from build123d import *

# Parameters (mm, degrees)
SKETCH_W        = 23
SKETCH_H        = 12
PAD_DEPTH       = 1
SKETCH001_W     = 4
SKETCH001_H     = 4
SKETCH001_W_2   = 9
SKETCH001_W_3   = 1.8
SKETCH001_H_2   = 2.119738
SKETCH001_W_4   = 1.7
SKETCH001_H_3   = 1.880262
SKETCH001_H_4   = 2.108956
SKETCH001_W_5   = 1.95
SKETCH001_H_5   = 1.880263
SKETCH001_H_6   = 2.119737
POCKET_DEPTH    = 5
SKETCH002_W     = 6
SKETCH002_H     = 12
POCKET001_DEPTH = 5


with BuildPart() as part:
    # Sketch → Pad (new body)
    with BuildSketch(Plane.XZ):
        with Locations((0.224666, -4.175566)):
            Rectangle(SKETCH_W, SKETCH_H)
    extrude(amount=PAD_DEPTH)

    # Sketch001 (on Face6 of Pad) → Pocket (cut)
    with BuildSketch(Plane.XZ.offset(1)):
        with Locations((-7.275334, -6.675566)):
            Rectangle(SKETCH001_W, SKETCH001_H)
        with Locations((7.724666, -6.675566)):
            Rectangle(SKETCH001_W, SKETCH001_H)
        with Locations((0.224666, -6.675566)):
            Rectangle(SKETCH001_W_2, SKETCH001_H)
        with Locations((-8.375334, -0.735435)):
            Rectangle(SKETCH001_W_3, SKETCH001_H_2)
        with Locations((-6.125334, -0.735435)):
            Rectangle(SKETCH001_W_4, SKETCH001_H_2)
        with Locations((-8.375334, -3.235435)):
            Rectangle(SKETCH001_W_3, SKETCH001_H_3)
        with Locations((-6.125334, -3.235435)):
            Rectangle(SKETCH001_W_4, SKETCH001_H_3)
        with Locations((-3.375334, -0.730044)):
            Rectangle(SKETCH001_W_3, SKETCH001_H_4)
        with Locations((-1.000334, -0.730044)):
            Rectangle(SKETCH001_W_5, SKETCH001_H_4)
        with Locations((-3.375334, -3.224654)):
            Rectangle(SKETCH001_W_3, SKETCH001_H_5)
        with Locations((-1.000334, -3.224654)):
            Rectangle(SKETCH001_W_5, SKETCH001_H_5)
        with Locations((1.374666, -0.730044)):
            Rectangle(SKETCH001_W_3, SKETCH001_H_4)
        with Locations((3.674666, -0.724653)):
            Rectangle(SKETCH001_W_3, SKETCH001_H_6)
        with Locations((1.374666, -3.224654)):
            Rectangle(SKETCH001_W_3, SKETCH001_H_5)
        with Locations((3.749666, -3.224654)):
            Rectangle(SKETCH001_W_5, SKETCH001_H_5)
        with Locations((6.624666, -0.732224)):
            Rectangle(SKETCH001_W_3, SKETCH001_H_2)
        with Locations((8.874666, -0.732224)):
            Rectangle(SKETCH001_W_4, SKETCH001_H_2)
        with Locations((6.624666, -3.232224)):
            Rectangle(SKETCH001_W_3, SKETCH001_H_3)
        with Locations((8.874666, -3.232224)):
            Rectangle(SKETCH001_W_4, SKETCH001_H_3)
    extrude(amount=-POCKET_DEPTH, mode=Mode.SUBTRACT)

    # Sketch002 (on Face5 of Pocket) → Pocket001 (cut)
    with BuildSketch(Plane.XZ.offset(1)):
        with Locations((-8.275334, -4.175566)):
            Rectangle(SKETCH002_W, SKETCH002_H)
        with Locations((8.724666, -4.175566)):
            Rectangle(SKETCH002_W, SKETCH002_H)
    extrude(amount=-POCKET001_DEPTH, mode=Mode.SUBTRACT)


solid = part.part
Work out the finished part from the listing and answer in its coordinate system (mm). A direction names the side the tool comes from. Round coordinates to 2 decimals unless told otherwise and drop trailing zeros. Write each loop counter-clockwise with the first axis right and the second up, starting at its lowest first coordinate (ties: lowest second). Pieces come first, ordered by that corner, then holes.
1) A cutting plane is placed at A-A (z = -2.75). Give the vertices of the cut face in (x, y).
2) A cutting plane is placed at D-D (z = -1). Give the vertices of the cut face in (x, y).
3) A tool of negligible diameter and unlimited length cuts with its end or side. For faces 3 (the flat face through (2.275, -0.5, -0.7)), 4 (the flat face through (5.725, -0.5, -4.3)), from which of +Z, -Z, +X, -X, +Y, -Y can it reach the whole face along a straight path? Write none if from no direction.
4) A cutting plane is placed at C-C (x = 1). Give the vertices of the cut face in (y, z).
5) Straight lines are drawn through the part: line 1 (X direction, y = -0.55, z = -2.75); line 2 (Z direction, x = 3.75, y = -0.85); line 3 (X direction, y = -0.35, z = -1.75). For each, find the intervals that lie inside material, in ascending order.
6) A cutting plane is placed at B-B (z = -7). Give the vertices of the cut face in (x, y).
7) The mould has two halves that part along Z. Classify faces 1 (the flat face through (4.725, -0.5, -6.7)), 2 (the flat face through (0.15, -1, -4.09)): pulls with the +Z half, pulls with the -Z half, needs draft (parallel to the pull), parting line crosses it, or undercut.
Completed:
1. outline: (-5.28, -1) - (-4.28, -1) - (-4.28, 0) - (-5.28, 0) - close; (-2.48, -1) - (-1.98, -1) - (-1.98, 0) - (-2.48, 0) - close; (-0.03, -1) - (0.47, -1) - (0.47, 0) - (-0.03, 0) - close; (2.27, -1) - (2.77, -1) - (2.77, 0) - (2.27, 0) - close; (4.72, -1) - (5.72, -1) - (5.72, 0) - (4.72, 0) - close
2. outline: (-5.28, -1) - (-4.28, -1) - (-4.28, 0) - (-5.28, 0) - close; (-2.48, -1) - (-1.98, -1) - (-1.98, 0) - (-2.48, 0) - close; (-0.03, -1) - (0.47, -1) - (0.47, 0) - (-0.03, 0) - close; (2.27, -1) - (2.77, -1) - (2.77, 0) - (2.27, 0) - close; (4.57, -1) - (5.72, -1) - (5.72, 0) - (4.57, 0) - close
3. face 3: +Y, -Y
3. face 4: +Z, -Z, +X, +Y, -Y
4. outline: (-1, -10.18) - (0, -10.18) - (0, -8.68) - (-1, -8.68) - close; (-1, -4.68) - (0, -4.68) - (0, -4.16) - (-1, -4.16) - close; (-1, -2.28) - (0, -2.28) - (0, -1.78) - (-1, -1.78) - close; (-1, 0.32) - (0, 0.32) - (0, 1.82) - (-1, 1.82) - close
5. line 1: x = -5.28 to -4.28, -2.48 to -1.98, -0.03 to 0.47, 2.27 to 2.77, 4.72 to 5.72
5. line 2: z = -10.18 to -8.68, -4.68 to -4.16, -2.28 to -1.78, 0.34 to 1.82
5. line 3: x = -5.28 to -4.28, -2.48 to -1.98, -0.03 to 0.47, 2.27 to 2.77, 4.57 to 5.72
6. outline: (-5.28, -1) - (-4.28, -1) - (-4.28, 0) - (-5.28, 0) - close; (4.72, -1) - (5.72, -1) - (5.72, 0) - (4.72, 0) - close
7. face 1: undercut
7. face 2: needs draft
